from build123d import *

# Parameters (mm, degrees)
BOSS_EXTRU_1_DEPTH      = 18
ENL_V_START             = -2
ESQUISSE2_W             = 17.221313325
ESQUISSE2_H             = 14
ENL_V_MAT_EXTRU_1_DEPTH = 30.036983947
D_GAGEMENT_M41_D        = 4.5
D_GAGEMENT_M42_D        = 4.5


with BuildPart() as part:
    # Esquisse1 → Boss.-Extru.1 (new body)
    with BuildSketch(Plane.XY):
        with BuildLine():
            Line((0, 1.5), (0, 16.378679656))
            ThreePointArc((0, 16.378679656), (-0.925974851, 17.764498955), (-2.560660172, 17.439339828))
            Line((-2.560660172, 17.439339828), (-17.439339828, 2.560660172))
            ThreePointArc((-17.439339828, 2.560660172), (-17.764498955, 0.925974851), (-16.378679656, 0))
            Line((-16.378679656, 0), (-1.5, 0))
            ThreePointArc((-1.5, 0), (-0.439339828, 0.439339828), (0, 1.5))
        make_face()
    extrude(amount=BOSS_EXTRU_1_DEPTH)

    # Esquisse2 → Enlèv. mat.-Extru.1 (cut, through all)
    with BuildSketch(Plane.XZ.offset(ENL_V_START)):
        with Locations((-10.610656663, 9)):
            Rectangle(ESQUISSE2_W, ESQUISSE2_H)
    extrude(amount=-ENL_V_MAT_EXTRU_1_DEPTH, mode=Mode.SUBTRACT)

    # Dégagement M41 (through all)
    with Locations(Plane(origin=(0, 0, 0), x_dir=(0, 0, -1), z_dir=(1, 0, 0))):
        with Locations((-9, 8.939339828)):
            Hole(D_GAGEMENT_M41_D / 2)

    # Dégagement M42 (through all)
    with Locations(Plane(origin=(0, 0, 0), x_dir=(-1, 0, 0), z_dir=(0, -1, 0))):
        with Locations((8.939339828, -9)):
            Hole(D_GAGEMENT_M42_D / 2)


solid = part.part
Source: CAD feature listing. Evaluate the final solid. Frame: model axes, mm. A direction names the side the tool comes from. Round coordinates to 2 decimals unless told otherwise and drop trailing zeros. Loops run counter-clockwise (first coordinate to the right, second up) from the corner with the lowest first, then second, coordinate; pieces in that order, holes last.
Q1. Ray query, line 1 (Y direction, x = -1.45, z = 9); line 2 (Z direction, x = -14, y = 3.25); line 3 (Y direction, x = -12.25, z = 9). Return the intervals inside material, ascending.
Q2. Mould query, pull axis Z, two halves, no side actions, for faces 3 (the face through (-8, 8, 2)), 4 (the face through (-10, 10, 1)), 5 (the face through (-7, 7, 0)). Classes: pulls with the +Z half, pulls with the -Z half, needs draft (parallel to the pull), parting line crosses it, or undercut.
Q3. Section D-D, the plane x = -13.25. Return loops of the section in (y, z), plus the area to 3 significant figures.
Q4. Section C-C, the plane y = 13.25. Return loops of the section in (x, z), plus the area to 3 significant figures.
Q5. First-contact query: P1, Ø1, axis at x = -9.5, z = 11.5, coming from the +Y side; P2, Ø2, axis at x = -8, z = 8, coming from the -Y side; P3, Ø3, axis at y = 4, z = 11.5, coming from the -X side; P4, Ø1, axis at x = -9.5, z = 9.5, coming from the -Y side. Flat tips, straight axial feed; report the tip coordinate or a pass-through.
Q6. Section A-A, the plane z = 9. Return loops of the section in (x, y), plus the area to 3 significant figures.
Q7. Section B-B, the plane x = -9. Return loops of the section in (y, z), plus the area to 3 significant figures.
Q8. Access query for faces 1 (the face through (-1.014, 9.038, 6.752)), 2 (the face through (-2, 12, 9)). Directions: +Z, -Z, +X, -X, +Y, -Y. A direction counts if a zero-diameter tool reaches every point of the face in a straight line with its end or side. Return the directions, or none.
Solutions:
1. line 1: y = 0 to 6.69, 11.19 to 17.88
1. line 2: z = 0 to 2, 16 to 18
1. line 3: y = 0 to 2
2. face 3: undercut
2. face 4: needs draft
2. face 5: pulls with the -Z half
3. outline: (0, 0) - (6.75, 0) - (6.75, 2) - (2, 2) - (2, 16) - (6.75, 16) - (6.75, 18) - (0, 18) - close
3. area: 55.0 mm2
4. outline: (-6.75, 0) - (0, 0) - (0, 18) - (-6.75, 18) - (-6.75, 16) - (-2, 16) - (-2, 2) - (-6.75, 2) - close
4. area: 55.0 mm2
5. P1: stops at y = 2
5. P2: stops at y = 0
5. P3: stops at x = -2
5. P4: passes through
6. outline: (-17.79, 2) arc R1.5 ccw to (-16.38, 0) - (-11.19, 0) - (-11.19, 2) - close; (-6.69, 0) - (-1.5, 0) arc R1.5 ccw to (0, 1.5) - (0, 6.69) - (-2, 6.69) - (-2, 2) - (-6.69, 2) - close; (-2, 11.19) - (0, 11.19) - (0, 16.38) arc R1.5 ccw to (-2, 17.79) - close
6. area: 48.0 mm2
7. outline: (0, 0) - (11, 0) - (11, 2) - (2, 2) - (2, 6.75) - (0, 6.75) - close; (0, 11.25) - (2, 11.25) - (2, 16) - (11, 16) - (11, 18) - (0, 18) - close
7. area: 63.0 mm2
8. face 1: +X, -X
8. face 2: -X, +Y
